```python
from build123d import *

# Parameters (mm, degrees)
F0_R     = 21.5
F1_DEPTH = 8
F2_R     = 19
F3_DEPTH = 8
F4_R     = 4
F5_R     = 5
F6_R     = 15
F7_DEPTH = 14


with BuildPart() as f1:
    # F0 (on Top) → F1 (new body)
    with BuildSketch(Plane.XY):
        Circle(F0_R)
    extrude(amount=F1_DEPTH)

    # F2 (on face) → F3 (join)
    with BuildSketch(Plane.XY.offset(8)):
        Circle(F2_R)
    extrude(amount=F3_DEPTH)

    # F4
    f4_edges = [f1.edges().sort_by_distance(p)[0] for p in [
        (-19, 0, 16),
    ]]
    fillet(f4_edges, radius=F4_R)

    # F5
    f5_edges = [f1.edges().sort_by_distance(p)[0] for p in [
        (-21.5, 0, 0),
    ]]
    fillet(f5_edges, radius=F5_R)

    # F6 (on face) → F7 (cut)
    with BuildSketch(Plane.XY.offset(16)):
        Circle(F6_R)
    extrude(amount=-F7_DEPTH, mode=Mode.SUBTRACT)


solid = f1.part
```
Could you check a few things on this model? Use its own coordinates, in mm. A direction names the side the tool comes from. Give positions to 0.01 mm unless a question says otherwise; leave off trailing zeros. Loops run counter-clockwise (first coordinate to the right, second up) from the corner with the lowest first, then second, coordinate; pieces in that order, holes last. Notation, with made-up numbers: (-28.75, -20.75) -> (11.25, -20.75) arc R16 cw to (11.25, 5.25) -> close; hole circle Ø4 at (87, 56.5). An arc over 180 degrees is marked (long way). Put each result on its own line as item: value.
(1) Imagine slicing it at A-A on y = 0. Write out the boundary of the cut face in (x, z).
Computed:
outline: (-21.5, 5) arc R5 ccw to (-16.5, 0) -> (16.5, 0) arc R5 ccw to (21.5, 5) -> (21.5, 8) -> (19, 8) -> (19, 12) arc R4 ccw to (15, 16) -> (15, 2) -> (-15, 2) -> (-15, 16) arc R4 ccw to (-19, 12) -> (-19, 8) -> (-21.5, 8) -> close
(2) For faces 1 (the face through (0, 0, 2)), 2 (the face through (0, 0, 0)), which set-ups out of +Z, -Z, +X, -X, +Y, -Y let a thin tool reach every point of the face, with its end or its side?
Computed:
face 1: +Z
face 2: -Z, +X, -X, +Y, -Y
(3) I'm going to push flat-ended pins straight in: pin 1 Ø10 at (x, y) = (-9.5, 1) entering from -Z; pin 2 Ø9 at (x, y) = (-4, 2.5) entering from +Z; pin 3 Ø5 at (x, z) = (-6, 10) entering from -Y; pin 4 Ø4 at (x, z) = (-1.5, 14) entering from +Y. Where does each tip first touch, or does it pass through?
Computed:
pin 1: z = 0
pin 2: z = 2
pin 3: y = -21.02
pin 4: y = 18.98
(4) Please list where these lines run through material, in increasing order: probe 1 along Y at (x, z) = (0, 12); probe 2 along Z at (x, y) = (11, -7.5); probe 3 along Y at (x, z) = (12, 13). Write a range as [from, to].
Computed:
probe 1: [-19, -15], [15, 19]
probe 2: [0, 2]
probe 3: [-14.57, -9], [9, 14.57]
(5) Thinking about a two-plate mould opening in Y: for faces 3 (the face through (-2.799, 21.317, 6.479)), 4 (the face through (11, -16, 8)), 5 (the face through (-14.985, 0.66, 9.098)), which applies, pulls with the +Y half, pulls with the -Y half, needs draft (parallel to the pull), parting line crosses it, or undercut?
Computed:
face 3: parting line crosses it
face 4: needs draft
face 5: undercut
(6) Imagine slicing it at C-C on z = 9.75. Write out the boundary of the cut face in (x, y), plus the area to 3 significant figures.
Computed:
outline: circle Ø38 at (0, 0); hole circle Ø30 at (0, 0)
area: 427 mm^2
(7) Imagine slicing it at D-D on z = 13.25. Write out the boundary of the cut face in (x, y), plus the area to 3 significant figures.
Computed:
outline: circle Ø37.6 at (0, 0); hole circle Ø30 at (0, 0)
area: 403 mm^2
